Read the model definition and answer for the solid it produces. Units are mm, in the model's axes. A direction names the side the tool comes from. Round coordinates to 2 decimals unless told otherwise and drop trailing zeros. Order: outer loops, then holes, each group sorted by start corner. A loop starts at its lowest first (then second) coordinate and runs counter-clockwise, first axis right, second up. Notation, with made-up numbers: M 46.25,8 L 53.25,8 A8 ccw 53.25,12 Z; hole C 14,-35 d8. An arc over 180 degrees is marked long. Answer as CSV lines item,"result".
```python
from build123d import *

# Parameters (mm, degrees)
SKETCH1_R           = 2.449
BOSS_EXTRUDE2_DEPTH = 2
BOSS_EXTRUDE3_DEPTH = 4


with BuildPart() as part:
    # Sketch1 → Boss-Extrude2 (new body)
    with BuildSketch(Plane.XY):
        with BuildLine():
            Line((9.168561928, 76.765332221), (-2.715276814, 76.765332221))
            ThreePointArc((-2.715276814, 76.765332221), (-5.543703939, 75.593759346), (-6.715276814, 72.765332221))
            Line((-6.715276814, 72.765332221), (-6.715276814, 32.85651365))
            ThreePointArc((-6.715276814, 32.85651365), (-5.543703939, 30.028086525), (-2.715276814, 28.85651365))
            Line((-2.715276814, 28.85651365), (81.739723186, 28.85651365))
            ThreePointArc((81.739723186, 28.85651365), (84.56815031, 30.028086525), (85.739723186, 32.85651365))
            Line((85.739723186, 32.85651365), (85.739723186, 72.765508714))
            ThreePointArc((85.739723186, 72.765508714), (84.56815031, 75.593935839), (81.739723186, 76.765508714))
            Line((81.739723186, 76.765508714), (70.033136805, 76.765508714))
            Line((70.033136805, 76.765508714), (9.168561928, 76.765332221))
        make_face()
        with Locations((50.884863874, 57.525313638)):
            Circle(SKETCH1_R, mode=Mode.SUBTRACT)
        with Locations((2.624863871, 57.525313638)):
            Circle(SKETCH1_R, mode=Mode.SUBTRACT)
        with BuildLine():
            Line((36.022761907, 69.590313638), (39.073863873, 69.590313638))
            ThreePointArc((39.073863873, 69.590313638), (42.306756076, 68.251205842), (43.645863873, 65.018313638))
            Line((43.645863873, 65.018313638), (43.645863873, 50.032313637))
            ThreePointArc((43.645863873, 50.032313637), (42.306756076, 46.799421434), (39.073863873, 45.460313637))
            Line((39.073863873, 45.460313637), (36.022761907, 45.460313637))
            Line((36.022761907, 45.460313637), (17.486965838, 45.460313637))
            Line((17.486965838, 45.460313637), (14.435863872, 45.460313637))
            ThreePointArc((14.435863872, 45.460313637), (11.202971669, 46.799421434), (9.863863872, 50.032313637))
            Line((9.863863872, 50.032313637), (9.863863872, 65.018313638))
            ThreePointArc((9.863863872, 65.018313638), (11.202971669, 68.251205842), (14.435863872, 69.590313638))
            Line((14.435863872, 69.590313638), (17.486965838, 69.590313638))
            Line((17.486965838, 69.590313638), (24.826000411, 69.590313638))
            Line((24.826000411, 69.590313638), (24.826000411, 70.340313638))
            Line((24.826000411, 70.340313638), (28.826000411, 70.340313638))
            Line((28.826000411, 70.340313638), (28.826000411, 69.590313638))
            Line((28.826000411, 69.590313638), (36.022761907, 69.590313638))
        make_face(mode=Mode.SUBTRACT)
    extrude(amount=BOSS_EXTRUDE2_DEPTH)

    # Sketch2 → Boss-Extrude3 (add)
    with BuildSketch(Plane(origin=(0, 0, 0), x_dir=(-1, 0, 0), z_dir=(0, 0, -1))):
        with BuildLine():
            Line((-83.439723186, 32.85651365), (-83.439723186, 35.85651365))
            Line((-83.439723186, 35.85651365), (-78.739723186, 31.15651365))
            Line((-78.739723186, 31.15651365), (-81.739723186, 31.15651365))
            ThreePointArc((-81.739723186, 31.15651365), (-82.941804714, 31.654432122), (-83.439723186, 32.85651365))
        make_face()
        with BuildLine():
            Line((-81.739723186, 74.465508714), (-78.739723186, 74.465508714))
            Line((-78.739723186, 74.465508714), (-83.439723186, 69.765508714))
            Line((-83.439723186, 69.765508714), (-83.439723186, 72.765508714))
            ThreePointArc((-83.439723186, 72.765508714), (-82.941804714, 73.967590242), (-81.739723186, 74.465508714))
        make_face()
        with BuildLine():
            Line((2.715276814, 31.15651365), (-0.284723186, 31.15651365))
            Line((-0.284723186, 31.15651365), (4.415276814, 35.85651365))
            Line((4.415276814, 35.85651365), (4.415276814, 32.85651365))
            ThreePointArc((4.415276814, 32.85651365), (3.917358342, 31.654432122), (2.715276814, 31.15651365))
        make_face()
        with BuildLine():
            Line((4.415276814, 72.765332221), (4.415276814, 69.765332221))
            Line((4.415276814, 69.765332221), (-0.284723186, 74.465332221))
            Line((-0.284723186, 74.465332221), (2.715276814, 74.465332221))
            ThreePointArc((2.715276814, 74.465332221), (3.917358342, 73.967413749), (4.415276814, 72.765332221))
        make_face()
    extrude(amount=BOSS_EXTRUDE3_DEPTH)


solid = part.part
```
Item 1: Flat-ended cylindrical pins translate along their axes: pin 1 (0.9 mm diameter, centred on x = 80.5, z = -2.5, fed in from +Y); pin 2 (24 mm diameter, centred on x = 16.5, y = 51.5, fed in from -Z); pin 3 (2.5 mm diameter, centred on y = 34.5, z = -1.5, fed in from +X). Find the tip coordinate at first contact, or state that the pin passes through.
Ans:
pin 1,"y = 74.47"
pin 2,"z = 0"
pin 3,"x = 83.44"
Item 2: A cutting plane is placed at C-C, the plane x = 13. Determine the outline of the cut face in (y, z).
Ans:
outline,"M 28.86,0 L 45.69,0 L 45.69,2 L 28.86,2 Z; M 69.36,0 L 76.77,0 L 76.77,2 L 69.36,2 Z"
Item 3: A tool of negligible diameter and unlimited length cuts with its end or side. For faces 1 (the face through (11.17, 68.22, 0.99)), 2 (the face through (81.123, 33.539, -1.972)), 3 (the face through (-4.415, 71, -2)), from which of +Z, -Z, +X, -X, +Y, -Y can it reach the whole face along a straight path? Write none if from no direction.
Ans:
face 1,"+Z, -Z"
face 2,"-Z"
face 3,"-Z, -X, +Y, -Y"
Item 4: A cutting plane is placed at D-D, the plane x = -1. Determine the outline of the cut face in (y, z), and give its area (3 significant figures).
Ans:
outline,"M 28.86,0 L 31.16,0 L 31.16,-4 L 32.44,-4 L 32.44,0 L 73.18,0 L 73.18,-4 L 74.47,-4 L 74.47,0 L 76.77,0 L 76.77,2 L 28.86,2 Z"
area,"106 mm2"
Item 5: A cutting plane is placed at A-A, the plane z = -2.2. Determine the outline of the cut face in (x, y), and give its area (3 significant figures).
Ans:
outline,"M -4.42,32.86 A1.7 ccw -2.72,31.16 L 0.28,31.16 L -4.42,35.86 Z; M -4.42,69.77 L 0.28,74.47 L -2.72,74.47 A1.7 ccw -4.42,72.77 Z; M 78.74,31.16 L 81.74,31.16 A1.7 ccw 83.44,32.86 L 83.44,35.86 Z; M 78.74,74.47 L 83.44,69.77 L 83.44,72.77 A1.7 ccw 81.74,74.47 Z"
area,"41.7 mm2"
Item 6: A cutting plane is placed at B-B, the plane y = 68.5. Determine the outline of the cut face in (x, z), and give its area (3 significant figures).
Ans:
outline,"M -6.72,0 L 11.47,0 L 11.47,2 L -6.72,2 Z; M 42.04,0 L 85.74,0 L 85.74,2 L 42.04,2 Z"
area,"124 mm2"
Item 7: Determine the mould class of faces 4 (the face through (84.54, 30, 0.99)), 5 (the face through (-1, 74.465, -2)), 6 (the face through (42.342, 46.835, 0.986)) for opening direction X: +X half, -X half, draft (parallel to the pull), parting line (faces both ways), or undercut.
Ans:
face 4,"+X half"
face 5,"draft"
face 6,"undercut"
Item 8: Find the intervals of material crossed by probe 1 along X at (y, z) = (56, 1.6); probe 2 along Y at (x, z) = (32, 0.1); probe 3 along X at (y, z) = (48, 1.75), in increasing order. Write a range as [from, to].
Ans:
probe 1,"[-6.72, 0.71], [4.54, 9.86], [43.65, 48.97], [52.8, 85.74]"
probe 2,"[28.86, 45.46], [69.59, 76.77]"
probe 3,"[-6.72, 10.34], [43.17, 85.74]"
